Answer from the drawing. Dimensions are ordinates in mm from the lowest x, y and z of the part. Round coordinates to 2 decimals unless told otherwise and drop trailing zeros. Loops run counter-clockwise (first coordinate to the right, second up) from the corner with the lowest first, then second, coordinate; pieces in that order, holes last. Notation, with made-up numbers: M 61.25,77.5 L 76.25,77.5 A17 ccw 76.25,96.5 Z; hole C 1,38 d6. An arc over 180 degrees is marked long. Write each question's results on one line, items separated by ' | '.
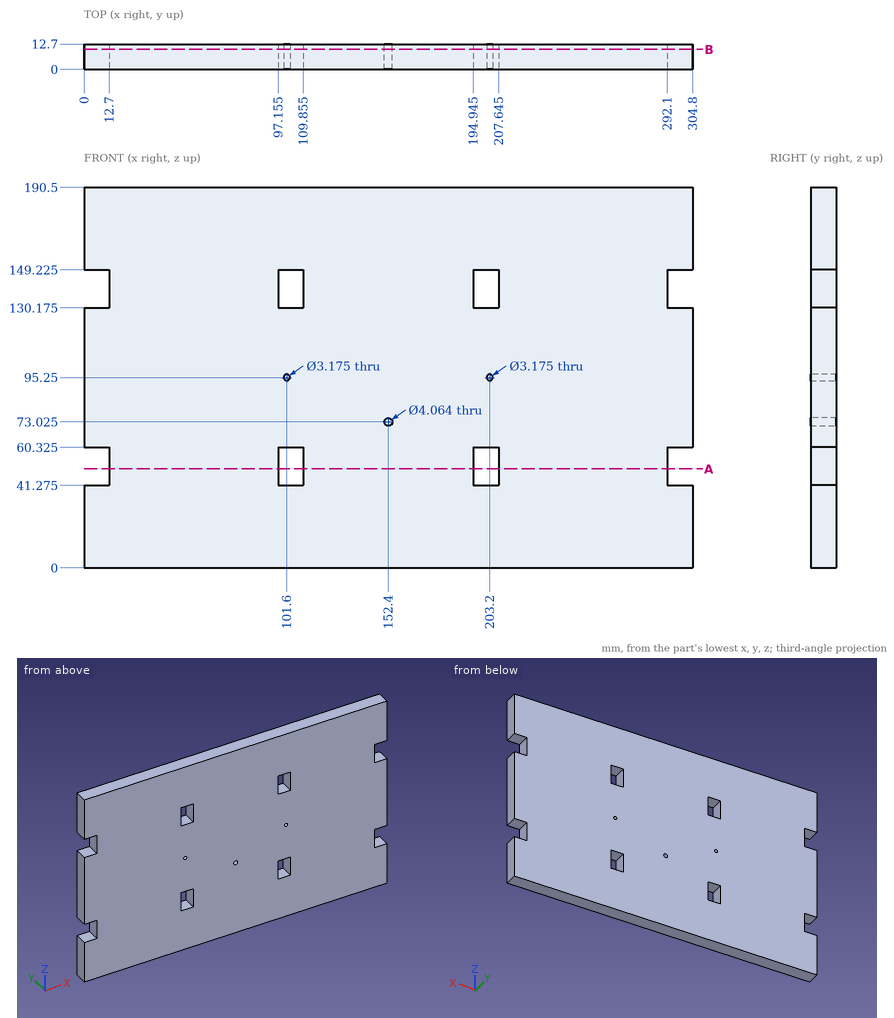
1. Given P1, Ø10, axis at x = 274, z = 34, coming from the -Y side; P2, Ø4, axis at y = 5.5, z = 141, coming from the -X side, each flat-ended and moving along its own axis, determine where each tip first touches the part or whether it passes through.
Completed:
P1: stops at y = 0 | P2: stops at x = 12.7
2. Find section A-A, the plane z = 49.5. Give the vertices of the cut face in (x, y) (3 decimals).
Completed:
outline: M 12.7,0 L 97.155,0 L 97.155,12.7 L 12.7,12.7 Z; M 109.855,0 L 194.945,0 L 194.945,12.7 L 109.855,12.7 Z; M 207.645,0 L 292.1,0 L 292.1,12.7 L 207.645,12.7 Z
3. Find the intervals of material crossed by L1, parallel to X at y = 4.75, z = 95.25; L2, parallel to Z at x = 203.2, y = 9.25 (1 decimal); L3, parallel to X at y = 3.5, z = 48.5 (3 decimals), in increasing order.
Completed:
L1: x = 0 to 100.01, 103.19 to 201.61, 204.79 to 304.8 | L2: z = 0 to 41.3, 60.3 to 93.7, 96.8 to 130.2, 149.2 to 190.5 | L3: x = 12.7 to 97.155, 109.855 to 194.945, 207.645 to 292.1
4. Find section B-B, the plane y = 10. Count the separate pieces of the cut face and the enclosed holes in it, then the cut area to 3 significant figures.
Completed:
separate pieces: 1 | enclosed holes: 7 | area: 56,100 mm2
